Input: dimensioned drawing with shaded views. Units: mm. Origin: part minimum x, y, z. Round coordinates to 2 decimals unless told otherwise and drop trailing zeros. Order: outer loops, then holes, each group sorted by start corner. A loop starts at its lowest first (then second) coordinate and runs counter-clockwise, first axis right, second up.
Item 1: Cut plane C-C on z = 4. Output: boundary loops of the cut face in (x, y).
Item 2: First-contact query: pin 1 (3 mm diameter, centred on x = 1.5, z = 4.5, fed in from -Y); pin 2 (3 mm diameter, centred on x = 17.5, z = 4.5, fed in from -Y); pin 3 (5 mm diameter, centred on x = 5, z = 7, fed in from +Y). Flat tips, straight axial feed; report the tip coordinate or a pass-through.
Item 3: Cut plane B-B on y = 16.25. Output: boundary loops of the cut face in (x, z).
Item 4: Cut plane D-D on x = 18. Output: boundary loops of the cut face in (y, z), then the cut area to 3 significant figures.
Item 5: Line query: L1, parallel to Z at x = 6.25, y = 13.5; L2, parallel to Y at x = 15.5, z = 8.5; L3, parallel to Y at x = 12.5, z = 4.25. Output: solid intervals per line, ascending.
Item 6: Cut plane A-A on x = 11.5. Output: boundary loops of the cut face in (y, z).
Item 7: Mould query, pull axis Y, two halves, no side actions, for the marked faces 1, 2 and 3. Classes: released by +Y, released by -Y, zero draft, split by the parting line, or undercut.
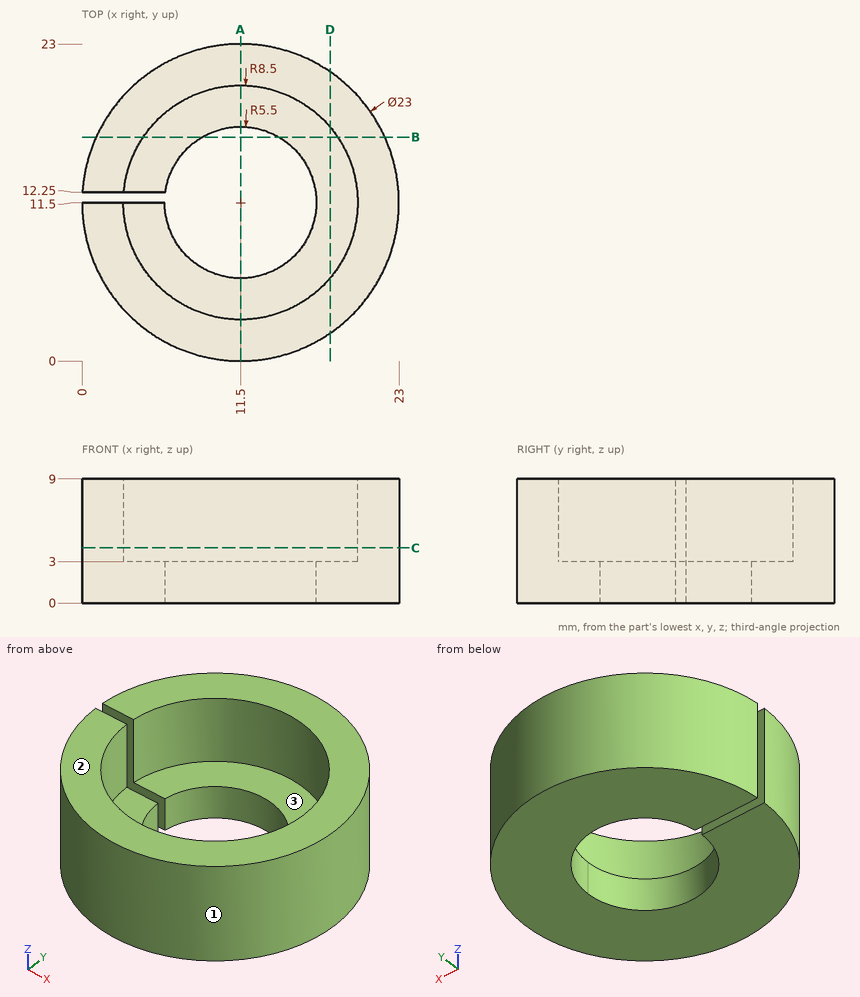
From the geometry:
1. outline: (0, 11.5) arc R11.5 ccw (long way) to (0.02, 12.25) - (3.03, 12.25) arc R8.5 cw (long way) to (3, 11.5) - close
2. pin 1: stops at y = 3.75
2. pin 2: stops at y = 0.92
2. pin 3: stops at y = 22.28
3. outline: (1.03, 0) - (8.73, 0) - (8.73, 3) - (4.45, 3) - (4.45, 9) - (1.03, 9) - close; (14.27, 0) - (21.97, 0) - (21.97, 9) - (18.55, 9) - (18.55, 3) - (14.27, 3) - close
4. outline: (2.01, 0) - (20.99, 0) - (20.99, 9) - (16.98, 9) - (16.98, 3) - (6.02, 3) - (6.02, 9) - (2.01, 9) - close
4. area: 105 mm2
5. L1: z = 0 to 3
5. L2: y = 0.72 to 4, 19 to 22.28
5. L3: y = 0.04 to 3.06, 19.94 to 22.96
6. outline: (0, 0) - (6, 0) - (6, 3) - (3, 3) - (3, 9) - (0, 9) - close; (17, 0) - (23, 0) - (23, 9) - (20, 9) - (20, 3) - (17, 3) - close
7. face 1: split by the parting line
7. face 2: zero draft
7. face 3: undercut
